Part print with two shaded views. Sizes in mm from the minimum x, y, z corner. A direction names the side the tool comes from. Give positions to 0.01 mm unless a question says otherwise; leave off trailing zeros. Loops run counter-clockwise (first coordinate to the right, second up) from the corner with the lowest first, then second, coordinate; pieces in that order, holes last. Notation, with made-up numbers: M 73,44.5 L 113,44.5 A21 cw 113,83.5 Z; hole C 29.5,-13.75 d5. An arc over 180 degrees is marked long. Answer as a JSON object with one key per item and string values. Group by question number.
1. Slice it at C-C (z = 26). List the corners of the cut face in (x, y), then the cut area to 3 significant figures.
2. Slice it at B-B (x = 262.5). List the corners of the cut face in (y, z).
3. Drop flat-ended pins along their axis: pin 1 Ø10 at (y, z) = (48, 21.5) entering from +X; pin 2 Ø12 at (x, z) = (50, 16.5) entering from +Y; pin 3 Ø21 at (y, z) = (54.5, 92) entering from -X; pin 4 Ø3 at (y, z) = (40, 18) entering from -X. Give the stop position or say it passes through.
4. Slice it at D-D (x = 195.5). List the corners of the cut face in (y, z), then the cut area to 3 significant figures.
5. Mould opens along X. For the marked faces 1, 2, 3 and 4 say: released by +X, released by -X, zero draft, split by the parting line, or undercut.
6. 3-axis set-ups, long thin cutter, end or side, ignore diameter. For the marked faces 5, 6 and 7: which of +Z, -Z, +X, -X, +Y, -Y reach the whole face in a straight line?
7. Drill centre lines: line 1 along Y through (x, z) = (119, 94.5); line 2 along Z through (x, y) = (136.5, 42); line 3 along Y through (x, z) = (237.5, 15.5). Where is each one in solid material? Low to high. Write a range as [from, to].
8. Slice it at A-A (z = 75). List the corners of the cut face in (x, y).
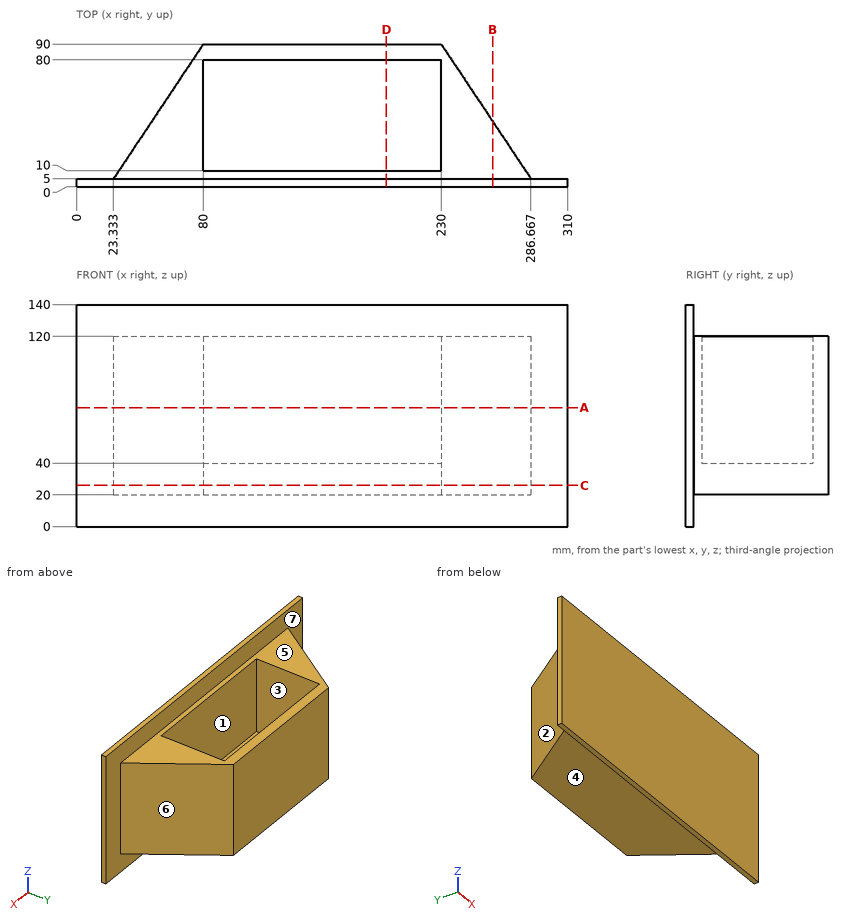
Established:
{
 "1": {"outline": "M 0,0 L 310,0 L 310,5 L 286.67,5 L 230,90 L 80,90 L 23.33,5 L 0,5 Z", "area": "19,100 mm^2"},
 "2": {"outline": "M 0,0 L 5,0 L 5,20 L 41.25,20 L 41.25,120 L 5,120 L 5,140 L 0,140 Z"},
 "3": {"pin 1": "stops at x = 261.33", "pin 2": "stops at y = 52.31", "pin 3": "stops at x = 49.33", "pin 4": "passes through"},
 "4": {"outline": "M 0,0 L 5,0 L 5,20 L 90,20 L 90,120 L 80,120 L 80,40 L 10,40 L 10,120 L 5,120 L 5,140 L 0,140 Z", "area": "3,600 mm^2"},
 "5": {"face 1": "undercut", "face 2": "released by -X", "face 3": "undercut", "face 4": "zero draft"},
 "6": {"face 5": "+Z, +X, -X, +Y", "face 6": "+Z, -Z, +X, +Y", "face 7": "+Y"},
 "7": {"line 1": "y = [0, 10], [80, 90]", "line 2": "z = [20, 40]", "line 3": "y = [0, 5]"},
 "8": {"outline": "M 0,0 L 310,0 L 310,5 L 286.67,5 L 230,90 L 80,90 L 23.33,5 L 0,5 Z; hole M 80,10 L 230,10 L 230,80 L 80,80 Z"}
}
